Source: CAD feature listing. Evaluate the final solid. Frame: model axes, mm. A direction names the side the tool comes from. Give positions to 0.01 mm unless a question says otherwise; leave off trailing zeros. Loops run counter-clockwise (first coordinate to the right, second up) from the corner with the lowest first, then second, coordinate; pieces in that order, holes last.
```python
from build123d import *

# Parameters (mm, degrees)
SKETCH1_W           = 50.8
SKETCH1_H           = 50.8
SKETCH1_W_2         = 44.45
BOSS_EXTRUDE1_DEPTH = 6.35
FILLET2_R           = 3.175
SKETCH2_R           = 6.35
BOSS_EXTRUDE3_DEPTH = 6.35
BOSS_EXTRUDE4_START = -6.35
SKETCH4_R           = 6.35
BOSS_EXTRUDE4_DEPTH = 6.35
CUT_EXTRUDE1_REACH  = 164.453
SKETCH2_4_R         = 4.49961
SKETCH2_4_R_2       = 1.9939


with BuildPart() as part:
    # Sketch1 → Boss-Extrude1 (new body)
    with BuildSketch(Plane(origin=(0, 0, 0), x_dir=(1, 0, 0), z_dir=(0, 1, 0))):
        Polygon((-146.05, 25.4), (-127, 25.4), (-127, -25.4), (-146.05, -25.4), (-146.05, -31.75), (146.05, -31.75), (146.05, -25.4), (127, -25.4), (127, 25.4), (146.05, 25.4), (146.05, 31.75), (-146.05, 31.75), align=None)
        with Locations((-31.75, 0)):
            Rectangle(SKETCH1_W, SKETCH1_H, mode=Mode.SUBTRACT)
        with Locations((-92.075, 0)):
            Rectangle(SKETCH1_W_2, SKETCH1_H, mode=Mode.SUBTRACT)
        with Locations((31.75, 0)):
            Rectangle(SKETCH1_W, SKETCH1_H, mode=Mode.SUBTRACT)
        with Locations((92.075, 0)):
            Rectangle(SKETCH1_W_2, SKETCH1_H, mode=Mode.SUBTRACT)
    extrude(amount=-BOSS_EXTRUDE1_DEPTH)

    # Fillet2
    fillet2_edges = [part.edges().sort_by_distance(p)[0] for p in [
        (-146.05, -6.35, 28.575),
        (-146.05, 0, 28.575),
        (-146.05, -6.35, -28.575),
        (-146.05, 0, -28.575),
        (146.05, -6.35, -28.575),
        (146.05, 0, -28.575),
        (146.05, -6.35, 28.575),
        (146.05, 0, 28.575),
    ]]
    fillet(fillet2_edges, radius=FILLET2_R - 0.0001)  # a hair under: the kernel refuses the full size

    # Sketch2 → Boss-Extrude3 (add)
    with BuildSketch(Plane.XY.offset(31.75)):
        with Locations((-142.875, -3.175)):
            Circle(SKETCH2_R)
    extrude(amount=-BOSS_EXTRUDE3_DEPTH)

    # Sketch4 → Boss-Extrude4 (add)
    with BuildSketch(Plane(origin=(0, 0, -31.75), x_dir=(-1, 0, 0), z_dir=(0, 0, -1)).offset(BOSS_EXTRUDE4_START)):
        with Locations((142.875, -3.175)):
            Circle(SKETCH4_R)
    extrude(amount=BOSS_EXTRUDE4_DEPTH)

    # Cut-Extrude1: up to this face of the body (flat: up to its plane)
    cut_extrude1_end = Plane(part.part.faces().sort_by_distance((-5.43222234, -3.175, -31.75))[0])
    # Sketch2<4> → Cut-Extrude1 (cut, up to the picked face)
    with BuildSketch(Plane.XY.offset(31.75), mode=Mode.PRIVATE) as cut_extrude1_sk1:
        with Locations((-142.875, -3.175)):
            Circle(SKETCH2_4_R)
    cut_extrude1_tool1 = split(extrude(cut_extrude1_sk1.sketch, amount=-CUT_EXTRUDE1_REACH, mode=Mode.PRIVATE), bisect_by=cut_extrude1_end, keep=Keep.BOTH, mode=Mode.PRIVATE)
    # Sketch2<4> → Cut-Extrude1 (cut, up to the picked face)
    with BuildSketch(Plane.XY.offset(31.75), mode=Mode.PRIVATE) as cut_extrude1_sk2:
        with Locations((-92.075, -3.175)):
            Circle(SKETCH2_4_R_2)
    cut_extrude1_tool2 = split(extrude(cut_extrude1_sk2.sketch, amount=-CUT_EXTRUDE1_REACH, mode=Mode.PRIVATE), bisect_by=cut_extrude1_end, keep=Keep.BOTH, mode=Mode.PRIVATE)
    # Sketch2<4> → Cut-Extrude1 (cut, up to the picked face)
    with BuildSketch(Plane.XY.offset(31.75), mode=Mode.PRIVATE) as cut_extrude1_sk3:
        with Locations((-31.75, -3.175)):
            Circle(SKETCH2_4_R_2)
    cut_extrude1_tool3 = split(extrude(cut_extrude1_sk3.sketch, amount=-CUT_EXTRUDE1_REACH, mode=Mode.PRIVATE), bisect_by=cut_extrude1_end, keep=Keep.BOTH, mode=Mode.PRIVATE)
    # Sketch2<4> → Cut-Extrude1 (cut, up to the picked face)
    with BuildSketch(Plane.XY.offset(31.75), mode=Mode.PRIVATE) as cut_extrude1_sk4:
        with Locations((31.75, -3.175)):
            Circle(SKETCH2_4_R_2)
    cut_extrude1_tool4 = split(extrude(cut_extrude1_sk4.sketch, amount=-CUT_EXTRUDE1_REACH, mode=Mode.PRIVATE), bisect_by=cut_extrude1_end, keep=Keep.BOTH, mode=Mode.PRIVATE)
    # Sketch2<4> → Cut-Extrude1 (cut, up to the picked face)
    with BuildSketch(Plane.XY.offset(31.75), mode=Mode.PRIVATE) as cut_extrude1_sk5:
        with Locations((92.075, -3.175)):
            Circle(SKETCH2_4_R_2)
    cut_extrude1_tool5 = split(extrude(cut_extrude1_sk5.sketch, amount=-CUT_EXTRUDE1_REACH, mode=Mode.PRIVATE), bisect_by=cut_extrude1_end, keep=Keep.BOTH, mode=Mode.PRIVATE)
    # Sketch2<4> → Cut-Extrude1 (cut, up to the picked face)
    with BuildSketch(Plane.XY.offset(31.75), mode=Mode.PRIVATE) as cut_extrude1_sk6:
        with Locations((-120.65, -3.175)):
            Circle(SKETCH2_4_R_2)
    cut_extrude1_tool6 = split(extrude(cut_extrude1_sk6.sketch, amount=-CUT_EXTRUDE1_REACH, mode=Mode.PRIVATE), bisect_by=cut_extrude1_end, keep=Keep.BOTH, mode=Mode.PRIVATE)
    # Sketch2<4> → Cut-Extrude1 (cut, up to the picked face)
    with BuildSketch(Plane.XY.offset(31.75), mode=Mode.PRIVATE) as cut_extrude1_sk7:
        with Locations((61.9125, -3.175)):
            Circle(SKETCH2_4_R_2)
    cut_extrude1_tool7 = split(extrude(cut_extrude1_sk7.sketch, amount=-CUT_EXTRUDE1_REACH, mode=Mode.PRIVATE), bisect_by=cut_extrude1_end, keep=Keep.BOTH, mode=Mode.PRIVATE)
    # Sketch2<4> → Cut-Extrude1 (cut, up to the picked face)
    with BuildSketch(Plane.XY.offset(31.75), mode=Mode.PRIVATE) as cut_extrude1_sk8:
        with BuildLine():
            Line((135.255, -1.1811), (142.875, -1.1811))
            ThreePointArc((142.875, -1.1811), (144.8689, -3.175), (142.875, -5.1689))
            Line((142.875, -5.1689), (135.255, -5.1689))
            ThreePointArc((135.255, -5.1689), (133.2611, -3.175), (135.255, -1.1811))
        make_face()
    cut_extrude1_tool8 = split(extrude(cut_extrude1_sk8.sketch, amount=-CUT_EXTRUDE1_REACH, mode=Mode.PRIVATE), bisect_by=cut_extrude1_end, keep=Keep.BOTH, mode=Mode.PRIVATE)
    add(cut_extrude1_tool1.solids().sort_by(Axis((-142.875, -3.175, 31.75), (0, 0, -1)))[0], mode=Mode.SUBTRACT)
    add(cut_extrude1_tool2.solids().sort_by(Axis((-92.075, -3.175, 31.75), (0, 0, -1)))[0], mode=Mode.SUBTRACT)
    add(cut_extrude1_tool3.solids().sort_by(Axis((-31.75, -3.175, 31.75), (0, 0, -1)))[0], mode=Mode.SUBTRACT)
    add(cut_extrude1_tool4.solids().sort_by(Axis((31.75, -3.175, 31.75), (0, 0, -1)))[0], mode=Mode.SUBTRACT)
    add(cut_extrude1_tool5.solids().sort_by(Axis((92.075, -3.175, 31.75), (0, 0, -1)))[0], mode=Mode.SUBTRACT)
    add(cut_extrude1_tool6.solids().sort_by(Axis((-120.65, -3.175, 31.75), (0, 0, -1)))[0], mode=Mode.SUBTRACT)
    add(cut_extrude1_tool7.solids().sort_by(Axis((61.9125, -3.175, 31.75), (0, 0, -1)))[0], mode=Mode.SUBTRACT)
    add(cut_extrude1_tool8.solids().sort_by(Axis((139.065, -3.175, 31.75), (0, 0, -1)))[0], mode=Mode.SUBTRACT)


solid = part.part
```
(1) Reachability of faces 4 (the flat face through (139, -1.181, 29)), 5 (the flat face through (134, -1, -25.4)), 6 (the flat face through (-32, -1, 25.4)) from +Z, -Z, +X, -X, +Y, -Y: full face, straight path, thin tool, end or side. Return the list, or none.
A:
face 4: +Z, -Z
face 5: +X, +Y, -Y
face 6: +Y, -Y
(2) First-contact query: pin 1 (4 mm diameter, centred on y = -2, z = -16.5, fed in from +X); pin 2 (3 mm diameter, centred on x = 62.5, z = -1.5, fed in from +Y); pin 3 (5 mm diameter, centred on y = -8, z = 13, fed in from -X). Flat tips, straight axial feed; report the tip coordinate or a pass-through.
A:
pin 1: stops at x = 127
pin 2: stops at y = 0
pin 3: stops at x = -127
(3) Section A-A, the plane x = 77. Return the cut outline in (y, z), then the cut area to 3 significant figures.
A:
outline: (-6.35, -31.75) - (0, -31.75) - (0, -25.4) - (-6.35, -25.4) - close; (-6.35, 25.4) - (0, 25.4) - (0, 31.75) - (-6.35, 31.75) - close
area: 80.6 mm2
(4) Ray query, line 1 along X through (y, z) = (-0.75, 20); line 2 along Z through (x, y) = (-84.5, -1.25); line 3 along Y through (x, z) = (119, -17). Return the intervals inside material, ascending.
A:
line 1: x = -127 to -114.3, -69.85 to -57.15, -6.35 to 6.35, 57.15 to 69.85, 114.3 to 127
line 2: z = -31.75 to -25.4, 25.4 to 31.75
line 3: y = -6.35 to 0
(5) Mould query, pull axis X, two halves, no side actions, for faces 1 (the cylindrical face through (-149.22, -2.94, 28.62)), 2 (the flat face through (69.85, -3, 0)), 3 (the flat face through (-127, -3, 0)). Classes: pulls with the +X half, pulls with the -X half, needs draft (parallel to the pull), parting line crosses it, or undercut.
A:
face 1: parting line crosses it
face 2: undercut
face 3: pulls with the -X half
(6) Section B-B, the plane z = 0. Count the separate pieces of the cut face and the enclosed holes in it, then the cut area to 3 significant figures.
A:
separate pieces: 5
enclosed holes: 2
area: 378 mm2
